Check sheet for the modelled part. Datum: model origin and axes. Units: mm. A direction names the side the tool comes from. Coordinates: 2 decimals unless noted, no trailing zeros. Order: outer loops, then holes, each group sorted by start corner. A loop starts at its lowest first (then second) coordinate and runs counter-clockwise, first axis right, second up. Notation, with made-up numbers: (-38, -33) -> (14, -33) arc R19 cw to (14, -21) -> close; hole circle Ø7 at (-37, -15). An arc over 180 degrees is marked (long way). Put each result on its own line as item: value. Start each with the question number.
```python
from build123d import *

# Parameters (mm, degrees)
SKETCH1_R           = 1.4
BOSS_EXTRUDE1_DEPTH = 2
SKETCH1_3_R         = 1.4
BOSS_EXTRUDE2_DEPTH = 10


with BuildPart() as part:
    # Sketch1 → Boss-Extrude1 (new body)
    with BuildSketch(Plane.XY):
        with BuildLine():
            ThreePointArc((-25, 12.25), (-23.828427125, 15.078427125), (-21, 16.25))
            Line((-21, 16.25), (21, 16.25))
            ThreePointArc((21, 16.25), (23.828427125, 15.078427125), (25, 12.25))
            Line((25, 12.25), (25, -12.25))
            ThreePointArc((25, -12.25), (23.828427125, -15.078427125), (21, -16.25))
            Line((21, -16.25), (-21, -16.25))
            ThreePointArc((-21, -16.25), (-23.828427125, -15.078427125), (-25, -12.25))
            Line((-25, -12.25), (-25, 12.25))
        make_face()
        with BuildLine():
            Line((-23, -12.25), (-23, 12.25))
            ThreePointArc((-23, 12.25), (-22.414213562, 13.664213562), (-21, 14.25))
            Line((-21, 14.25), (21, 14.25))
            ThreePointArc((21, 14.25), (22.414213562, 13.664213562), (23, 12.25))
            Line((23, 12.25), (23, -12.25))
            ThreePointArc((23, -12.25), (22.414213562, -13.664213562), (21, -14.25))
            Line((21, -14.25), (-21, -14.25))
            ThreePointArc((-21, -14.25), (-22.414213562, -13.664213562), (-23, -12.25))
        make_face(mode=Mode.SUBTRACT)
        with BuildLine():
            ThreePointArc((-23, 12.25), (-22.414213562, 13.664213562), (-21, 14.25))
            Line((-21, 14.25), (21, 14.25))
            ThreePointArc((21, 14.25), (22.414213562, 13.664213562), (23, 12.25))
            Line((23, 12.25), (23, -12.25))
            ThreePointArc((23, -12.25), (22.414213562, -13.664213562), (21, -14.25))
            Line((21, -14.25), (-21, -14.25))
            ThreePointArc((-21, -14.25), (-22.414213562, -13.664213562), (-23, -12.25))
            Line((-23, -12.25), (-23, 12.25))
        make_face()
        with BuildLine():
            Line((-22.5, -12.25), (-22.5, 12.25))
            ThreePointArc((-22.5, 12.25), (-22.060660172, 13.310660172), (-21, 13.75))
            Line((-21, 13.75), (21, 13.75))
            ThreePointArc((21, 13.75), (22.060660172, 13.310660172), (22.5, 12.25))
            Line((22.5, 12.25), (22.5, -12.25))
            ThreePointArc((22.5, -12.25), (22.060660172, -13.310660172), (21, -13.75))
            Line((21, -13.75), (-21, -13.75))
            ThreePointArc((-21, -13.75), (-22.060660172, -13.310660172), (-22.5, -12.25))
        make_face(mode=Mode.SUBTRACT)
        with BuildLine():
            ThreePointArc((-22.5, 12.25), (-22.060660172, 13.310660172), (-21, 13.75))
            Line((-21, 13.75), (21, 13.75))
            ThreePointArc((21, 13.75), (22.060660172, 13.310660172), (22.5, 12.25))
            Line((22.5, 12.25), (22.5, -12.25))
            ThreePointArc((22.5, -12.25), (22.060660172, -13.310660172), (21, -13.75))
            Line((21, -13.75), (-21, -13.75))
            ThreePointArc((-21, -13.75), (-22.060660172, -13.310660172), (-22.5, -12.25))
            Line((-22.5, -12.25), (-22.5, 12.25))
        make_face()
        with Locations((15, -8.1)):
            Circle(SKETCH1_R, mode=Mode.SUBTRACT)
        with Locations((-15, 8.1)):
            Circle(SKETCH1_R, mode=Mode.SUBTRACT)
        with Locations((15, -8.1)):
            Circle(SKETCH1_R)
        with Locations((-15, 8.1)):
            Circle(SKETCH1_R)
    extrude(amount=BOSS_EXTRUDE1_DEPTH)

    # Sketch1_3 → Boss-Extrude2 (add)
    with BuildSketch(Plane.XY):
        with BuildLine():
            ThreePointArc((-23, 12.25), (-22.414213562, 13.664213562), (-21, 14.25))
            Line((-21, 14.25), (21, 14.25))
            ThreePointArc((21, 14.25), (22.414213562, 13.664213562), (23, 12.25))
            Line((23, 12.25), (23, -12.25))
            ThreePointArc((23, -12.25), (22.414213562, -13.664213562), (21, -14.25))
            Line((21, -14.25), (-21, -14.25))
            ThreePointArc((-21, -14.25), (-22.414213562, -13.664213562), (-23, -12.25))
            Line((-23, -12.25), (-23, 12.25))
        make_face()
        with BuildLine():
            Line((-22.5, -12.25), (-22.5, 12.25))
            ThreePointArc((-22.5, 12.25), (-22.060660172, 13.310660172), (-21, 13.75))
            Line((-21, 13.75), (21, 13.75))
            ThreePointArc((21, 13.75), (22.060660172, 13.310660172), (22.5, 12.25))
            Line((22.5, 12.25), (22.5, -12.25))
            ThreePointArc((22.5, -12.25), (22.060660172, -13.310660172), (21, -13.75))
            Line((21, -13.75), (-21, -13.75))
            ThreePointArc((-21, -13.75), (-22.060660172, -13.310660172), (-22.5, -12.25))
        make_face(mode=Mode.SUBTRACT)
        with Locations((15, -8.1)):
            Circle(SKETCH1_3_R)
        with Locations((-15, 8.1)):
            Circle(SKETCH1_3_R)
    extrude(amount=BOSS_EXTRUDE2_DEPTH)


solid = part.part
```
1) Mould release check, pull along X, two halves, no side actions. Record for faces 6 (the cylindrical face through (22.07, -13.3, 5.94)), 7 (the cylindrical face through (-23.797, -15.109, 0.986)), 8 (the flat face through (0, 14.25, 6)), 9 (the cylindrical face through (22.05, 13.32, 5.94)): +X half, -X half, draft (parallel to the pull), parting line (faces both ways), or undercut.
2) Sectioned sample at A-A (z = 3.25). Record the boundary of the cut face in (x, y).
3) Access from +Z, -Z, +X, -X, +Y, -Y to the whole of each face (thin tool, end or side, straight path). Record for faces 1 (the flat face through (0, 0, 0)), 2 (the flat face through (0, -14.25, 6)), 3 (the flat face through (-23, 0, 6)), 4 (the flat face through (22.5, 0, 6)), 5 (the cylindrical face through (22.4, 13.68, 5.94)).
4) Gauge pin test, flat ends, axial feed: pin 1 (3 mm diameter, centred on x = -19.5, y = -10.5, fed in from +Z); pin 2 (2.5 mm diameter, centred on y = 0.5, z = 7.5, fed in from +X); pin 3 (2.5 mm diameter, centred on y = 3.5, z = 4.5, fed in from -X). Record the tip position at first contact, or that the pin passes through.
5) Sectioned sample at D-D (x = -9.5). Record the boundary of the cut face in (y, z).
6) Sectioned sample at C-C (y = -8.1). Record the boundary of the cut face in (x, z), plus the area to 3 significant figures.
7) Scan lines: line 1 along X through (y, z) = (8, 6.5); line 2 along Y through (x, z) = (-7.5, 4); line 3 along X through (y, z) = (-1.5, 9). Record each from-to range of solid material in increasing order. Write a range as [from, to].
8) Sectioned sample at B-B (x = -15). Record the boundary of the cut face in (y, z), plus the area to 3 significant figures.
Entries:
1. face 6: undercut
1. face 7: -X half
1. face 8: draft
1. face 9: undercut
2. outline: (-23, -12.25) arc R2 ccw to (-21, -14.25) -> (21, -14.25) arc R2 ccw to (23, -12.25) -> (23, 12.25) arc R2 ccw to (21, 14.25) -> (-21, 14.25) arc R2 ccw to (-23, 12.25) -> close; circle Ø2.8 at (-15, 8.1); circle Ø2.8 at (15, -8.1); hole (-22.5, -12.25) arc R1.5 ccw to (-21, -13.75) -> (21, -13.75) arc R1.5 ccw to (22.5, -12.25) -> (22.5, 12.25) arc R1.5 ccw to (21, 13.75) -> (-21, 13.75) arc R1.5 ccw to (-22.5, 12.25) -> close
3. face 1: -Z, +X, -X, +Y, -Y
3. face 2: +Z, +X, -X, -Y
3. face 3: +Z, -X, +Y, -Y
3. face 4: +Z
3. face 5: +Z, +X, +Y
4. pin 1: stops at z = 2
4. pin 2: stops at x = 23
4. pin 3: stops at x = -23
5. outline: (-16.25, 0) -> (16.25, 0) -> (16.25, 2) -> (14.25, 2) -> (14.25, 10) -> (13.75, 10) -> (13.75, 2) -> (-13.75, 2) -> (-13.75, 10) -> (-14.25, 10) -> (-14.25, 2) -> (-16.25, 2) -> close
6. outline: (-25, 0) -> (25, 0) -> (25, 2) -> (23, 2) -> (23, 10) -> (22.5, 10) -> (22.5, 2) -> (16.4, 2) -> (16.4, 10) -> (13.6, 10) -> (13.6, 2) -> (-22.5, 2) -> (-22.5, 10) -> (-23, 10) -> (-23, 2) -> (-25, 2) -> close
6. area: 130 mm2
7. line 1: x = [-23, -22.5], [-16.4, -13.6], [22.5, 23]
7. line 2: y = [-14.25, -13.75], [13.75, 14.25]
7. line 3: x = [-23, -22.5], [22.5, 23]
8. outline: (-16.25, 0) -> (16.25, 0) -> (16.25, 2) -> (14.25, 2) -> (14.25, 10) -> (13.75, 10) -> (13.75, 2) -> (9.5, 2) -> (9.5, 10) -> (6.7, 10) -> (6.7, 2) -> (-13.75, 2) -> (-13.75, 10) -> (-14.25, 10) -> (-14.25, 2) -> (-16.25, 2) -> close
8. area: 95.4 mm2
